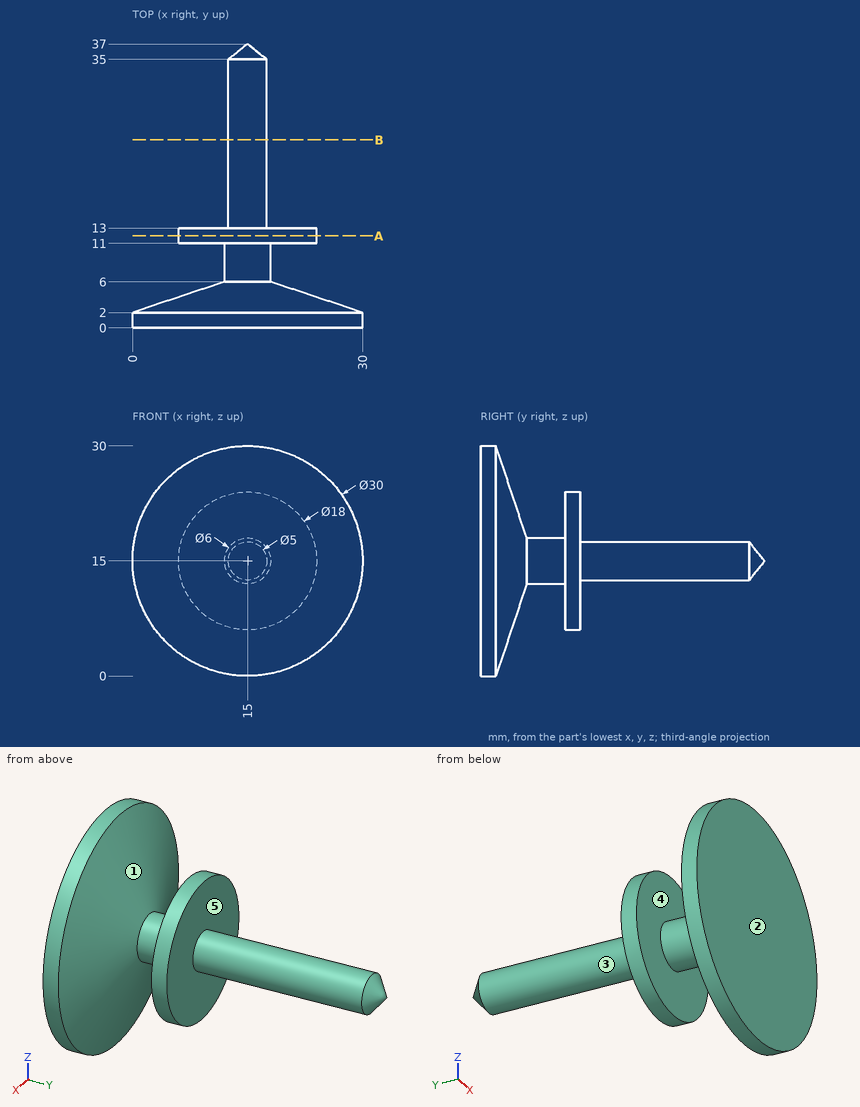
The drawing under review shows one solid part. Ordinate dimensions are in mm from its lowest x, y, z. A direction names the side the tool comes from. Coordinates: 2 decimals unless noted, no trailing zeros. Write each loop counter-clockwise with the first axis right and the second up, starting at its lowest first coordinate (ties: lowest second). Pieces come first, ordered by that corner, then holes. Notation, with made-up numbers: (60.5, 83) - (109.5, 83) arc R7 ccw to (109.5, 96) - close; hole circle Ø5 at (7.25, 83.25). An arc over 180 degrees is marked (long way). Answer in a Markdown table with one row per item. Add a question column.
Q1. Draft analysis for pull direction Y (two halves, no side actions). For the marked faces 3, 4 and 5, state which applies: +Y half, -Y half, draft (parallel to the pull), parting line (faces both ways), or undercut.
Q2. We need section B-B, the plane y = 24.5. State the section outline as (x, z) points, and give its area (3 significant figures).
Q3. For P1, Ø5.5, axis at x = 17.5, z = 18.5, coming from the +Y side; P2, Ø4, axis at x = 13, y = 30.5, coming from the +Z side; P3, Ø10, axis at y = 24.5, z = 18.5, coming from the +X side, all flat-tipped, find the tip position at first contact; note any pin that passes through.
Q4. For probe 1 along Y at (x, z) = (18.5, 10.75); probe 2 along Z at (x, y) = (15, 31.5); probe 3 along Y at (x, z) = (22.5, 11.5), list the stretches that pass through material, from the lowest coordinate up.
Q5. Tool access review of the marked faces 1 and 2: name each direction out of +Z, -Z, +X, -X, +Y, -Y from which nothing blocks a thin tool from reaching the whole face with its end or side.
Q6. We need section A-A, the plane y = 12. State the section outline as (x, z) points, and give its area (3 significant figures).
Answer list:
| question | item | result |
|---|---|---|
| 1 | face 3 | draft |
| 1 | face 4 | undercut |
| 1 | face 5 | +Y half |
| 2 | outline | circle Ø5 at (15, 15) |
| 2 | area | 19.6 mm2 |
| 3 | P1 | stops at y = 35.76 |
| 3 | P2 | stops at z = 17.5 |
| 3 | P3 | stops at x = 17.5 |
| 4 | probe 1 | y = 0 to 5.16, 11 to 13 |
| 4 | probe 2 | z = 12.5 to 17.5 |
| 4 | probe 3 | y = 0 to 4.24, 11 to 13 |
| 5 | face 1 | none |
| 5 | face 2 | +Z, -Z, +X, -X, -Y |
| 6 | outline | circle Ø18 at (15, 15) |
| 6 | area | 254 mm2 |
